Geometry check sheet. Reference: the model listing, model coordinates, mm. Face numbers are marked on the shaded views. A direction names the side the tool comes from. Give positions to 0.01 mm unless a question says otherwise; leave off trailing zeros. Write each loop counter-clockwise with the first axis right and the second up, starting at its lowest first coordinate (ties: lowest second). Pieces come first, ordered by that corner, then holes. Notation, with made-up numbers: M -25,51 L -13,51 A19 cw -13,58 Z; hole C -6.5,78.5 d5. An arc over 180 degrees is marked long. One line per item, written item: value. Start each with the question number.
1. Gauge pin test, flat ends, axial feed: pin 1 (3 mm diameter, centred on x = -74, z = -31.5, fed in from -Y); pin 2 (6 mm diameter, centred on x = -20, z = 45, fed in from +Y); pin 3 (6.5 mm diameter, centred on x = -40, z = 45.5, fed in from -Y); pin 4 (4 mm diameter, centred on x = 100, z = 45, fed in from +Y). Record the tip position at first contact, or that the pin passes through.
2. Cross-section at A-A on z = -45. Count the separate pieces of the cut face and the enclosed holes in it, then the cut area to 3 significant figures.
3. Cross-section at B-B on x = -51.5. Record the cut outline in (y, z).
4. Cross-section at C-C on z = 20. Record the cut outline in (x, y).
5. Tool access check on the marked faces 1 and 2. Record the directions out of +Z, -Z, +X, -X, +Y, -Y that give a thin tool (end or side, any length) a straight path to the whole face; none if there is none.
6. Release check for a two-part mould opening along Z. For the marked faces 3, 4 and 5 record: pulls with the +Z half, pulls with the -Z half, needs draft (parallel to the pull), parting line crosses it, or undercut.
7. Scan lines: line 1 (Z direction, x = -100, y = 9); line 2 (Z direction, x = 62, y = 9); line 3 (Z direction, x = 72.5, y = 7.5). Record each from-to range of solid material in increasing order.
from build123d import *

# Parameters (mm, degrees)
SKETCH2_W           = 240
SKETCH2_H           = 100
BOSS_EXTRUDE1_DEPTH = 12
HOLE1_AT_2_COUNT    = 2
HOLE1_AT_2_PITCH    = 228
SKETCH10_W          = 216
SKETCH10_H          = 76
CUT_EXTRUDE2_DEPTH  = 8
EXTRUDE_THIN1_DEPTH = 8
FILLET1_R           = 1


# Read off the part's stored shape, not the designer's step: CBORE for M4 SHCS1
with BuildPart() as part:
    # Sketch2 → Boss-Extrude1 (new body)
    with BuildSketch(Plane(origin=(0, 0, 0), x_dir=(1, 0, 0), z_dir=(0, 1, 0))):
        Rectangle(SKETCH2_W, SKETCH2_H)
    extrude(amount=BOSS_EXTRUDE1_DEPTH)

    # Sketch6 → Hole1 (revolve, cut)
    with BuildSketch(Plane(origin=(-114, 6, 50), x_dir=(0, -1, 0), z_dir=(1, 0, 0))):
        Polygon((0, 0), (0, 12), (1.85, 10.15), (1.85, 0), align=None)
    hole1 = revolve(axis=Axis((-114, 6, 54.244199587), (0, 0, -1)), mode=Mode.SUBTRACT)

    # Hole1 at 2: Hole1 ×2
    with Locations(*[(i * HOLE1_AT_2_PITCH, 0, 0) for i in range(1, HOLE1_AT_2_COUNT)]):
        add(hole1, mode=Mode.SUBTRACT)

    # Mirror2: Hole1 across plane
    add(hole1.mirror(Plane.XY), mode=Mode.SUBTRACT)

    # Mirror2 copy 1 sketch → Mirror2 copy 1 (revolve, cut)
    with BuildSketch(Plane(origin=(114, 6, -50), x_dir=(0, -1, 0), z_dir=(1, 0, 0))):
        Polygon((0, 0), (0, -12), (1.85, -10.15), (1.85, 0), align=None)
    revolve(axis=Axis((114, 6, -54.244199587), (0, 0, -1)), mode=Mode.SUBTRACT)

    # CBORE for M4 SHCS1 outline → CBORE for M4 SHCS1 (revolve, cut)
    with BuildSketch(Plane(origin=(-100, 0, -45), x_dir=(1, 0, 0), z_dir=(0, 0, 1))):
        Polygon((2.25, 4), (2.25, 12), (0, 12), (0, 0), (4.025, 0), (4, 0.025), (4, 4), align=None)
    revolve(axis=Axis((-100, 0, -45), (0, 1, 0)), mode=Mode.SUBTRACT)

    # CBORE for M4 SHCS1 2 outline → CBORE for M4 SHCS1 2 (revolve, cut)
    with BuildSketch(Plane(origin=(-100, 0, 45), x_dir=(1, 0, 0), z_dir=(0, 0, 1))):
        Polygon((0, 0), (4.025, 0), (4, 0.025), (4, 4), (2.25, 4), (2.25, 12), (0, 12), align=None)
    revolve(axis=Axis((-100, 0, 45), (0, 1, 0)), mode=Mode.SUBTRACT)

    # CBORE for M4 SHCS1 3 outline → CBORE for M4 SHCS1 3 (revolve, cut)
    with BuildSketch(Plane(origin=(-80, 0, -45), x_dir=(1, 0, 0), z_dir=(0, 0, 1))):
        Polygon((0, 0), (4.025, 0), (4, 0.025), (4, 4), (2.25, 4), (2.25, 12), (0, 12), align=None)
    revolve(axis=Axis((-80, 0, -45), (0, 1, 0)), mode=Mode.SUBTRACT)

    # CBORE for M4 SHCS1 4 outline → CBORE for M4 SHCS1 4 (revolve, cut)
    with BuildSketch(Plane(origin=(-80, 0, 45), x_dir=(1, 0, 0), z_dir=(0, 0, 1))):
        Polygon((0, 0), (4.025, 0), (4, 0.025), (4, 4), (2.25, 4), (2.25, 12), (0, 12), align=None)
    revolve(axis=Axis((-80, 0, 45), (0, 1, 0)), mode=Mode.SUBTRACT)

    # CBORE for M4 SHCS1 5 outline → CBORE for M4 SHCS1 5 (revolve, cut)
    with BuildSketch(Plane(origin=(-60, 0, -45), x_dir=(1, 0, 0), z_dir=(0, 0, 1))):
        Polygon((0, 0), (4.025, 0), (4, 0.025), (4, 4), (2.25, 4), (2.25, 12), (0, 12), align=None)
    revolve(axis=Axis((-60, 0, -45), (0, 1, 0)), mode=Mode.SUBTRACT)

    # CBORE for M4 SHCS1 6 outline → CBORE for M4 SHCS1 6 (revolve, cut)
    with BuildSketch(Plane(origin=(-60, 0, 45), x_dir=(1, 0, 0), z_dir=(0, 0, 1))):
        Polygon((0, 0), (4.025, 0), (4, 0.025), (4, 4), (2.25, 4), (2.25, 12), (0, 12), align=None)
    revolve(axis=Axis((-60, 0, 45), (0, 1, 0)), mode=Mode.SUBTRACT)

    # CBORE for M4 SHCS1 7 outline → CBORE for M4 SHCS1 7 (revolve, cut)
    with BuildSketch(Plane(origin=(-40, 0, -45), x_dir=(1, 0, 0), z_dir=(0, 0, 1))):
        Polygon((0, 0), (4.025, 0), (4, 0.025), (4, 4), (2.25, 4), (2.25, 12), (0, 12), align=None)
    revolve(axis=Axis((-40, 0, -45), (0, 1, 0)), mode=Mode.SUBTRACT)

    # CBORE for M4 SHCS1 8 outline → CBORE for M4 SHCS1 8 (revolve, cut)
    with BuildSketch(Plane(origin=(-40, 0, 45), x_dir=(1, 0, 0), z_dir=(0, 0, 1))):
        Polygon((0, 0), (4.025, 0), (4, 0.025), (4, 4), (2.25, 4), (2.25, 12), (0, 12), align=None)
    revolve(axis=Axis((-40, 0, 45), (0, 1, 0)), mode=Mode.SUBTRACT)

    # CBORE for M4 SHCS1 9 outline → CBORE for M4 SHCS1 9 (revolve, cut)
    with BuildSketch(Plane(origin=(-20, 0, -45), x_dir=(1, 0, 0), z_dir=(0, 0, 1))):
        Polygon((0, 0), (4.025, 0), (4, 0.025), (4, 4), (2.25, 4), (2.25, 12), (0, 12), align=None)
    revolve(axis=Axis((-20, 0, -45), (0, 1, 0)), mode=Mode.SUBTRACT)

    # CBORE for M4 SHCS1 10 outline → CBORE for M4 SHCS1 10 (revolve, cut)
    with BuildSketch(Plane(origin=(-20, 0, 45), x_dir=(1, 0, 0), z_dir=(0, 0, 1))):
        Polygon((0, 0), (4.025, 0), (4, 0.025), (4, 4), (2.25, 4), (2.25, 12), (0, 12), align=None)
    revolve(axis=Axis((-20, 0, 45), (0, 1, 0)), mode=Mode.SUBTRACT)

    # CBORE for M4 SHCS1 11 outline → CBORE for M4 SHCS1 11 (revolve, cut)
    with BuildSketch(Plane.XY.offset(-45)):
        Polygon((0, 0), (4.025, 0), (4, 0.025), (4, 4), (2.25, 4), (2.25, 12), (0, 12), align=None)
    revolve(axis=Axis((0, 0, -45), (0, 1, 0)), mode=Mode.SUBTRACT)

    # CBORE for M4 SHCS1 12 outline → CBORE for M4 SHCS1 12 (revolve, cut)
    with BuildSketch(Plane.XY.offset(45)):
        Polygon((0, 0), (4.025, 0), (4, 0.025), (4, 4), (2.25, 4), (2.25, 12), (0, 12), align=None)
    revolve(axis=Axis((0, 0, 45), (0, 1, 0)), mode=Mode.SUBTRACT)

    # CBORE for M4 SHCS1 13 outline → CBORE for M4 SHCS1 13 (revolve, cut)
    with BuildSketch(Plane(origin=(20, 0, -45), x_dir=(1, 0, 0), z_dir=(0, 0, 1))):
        Polygon((0, 0), (4.025, 0), (4, 0.025), (4, 4), (2.25, 4), (2.25, 12), (0, 12), align=None)
    revolve(axis=Axis((20, 0, -45), (0, 1, 0)), mode=Mode.SUBTRACT)

    # CBORE for M4 SHCS1 14 outline → CBORE for M4 SHCS1 14 (revolve, cut)
    with BuildSketch(Plane(origin=(20, 0, 45), x_dir=(1, 0, 0), z_dir=(0, 0, 1))):
        Polygon((0, 0), (4.025, 0), (4, 0.025), (4, 4), (2.25, 4), (2.25, 12), (0, 12), align=None)
    revolve(axis=Axis((20, 0, 45), (0, 1, 0)), mode=Mode.SUBTRACT)

    # CBORE for M4 SHCS1 15 outline → CBORE for M4 SHCS1 15 (revolve, cut)
    with BuildSketch(Plane(origin=(40, 0, -45), x_dir=(1, 0, 0), z_dir=(0, 0, 1))):
        Polygon((0, 0), (4.025, 0), (4, 0.025), (4, 4), (2.25, 4), (2.25, 12), (0, 12), align=None)
    revolve(axis=Axis((40, 0, -45), (0, 1, 0)), mode=Mode.SUBTRACT)

    # CBORE for M4 SHCS1 16 outline → CBORE for M4 SHCS1 16 (revolve, cut)
    with BuildSketch(Plane(origin=(40, 0, 45), x_dir=(1, 0, 0), z_dir=(0, 0, 1))):
        Polygon((0, 0), (4.025, 0), (4, 0.025), (4, 4), (2.25, 4), (2.25, 12), (0, 12), align=None)
    revolve(axis=Axis((40, 0, 45), (0, 1, 0)), mode=Mode.SUBTRACT)

    # CBORE for M4 SHCS1 17 outline → CBORE for M4 SHCS1 17 (revolve, cut)
    with BuildSketch(Plane(origin=(60, 0, -45), x_dir=(1, 0, 0), z_dir=(0, 0, 1))):
        Polygon((0, 0), (4.025, 0), (4, 0.025), (4, 4), (2.25, 4), (2.25, 12), (0, 12), align=None)
    revolve(axis=Axis((60, 0, -45), (0, 1, 0)), mode=Mode.SUBTRACT)

    # CBORE for M4 SHCS1 18 outline → CBORE for M4 SHCS1 18 (revolve, cut)
    with BuildSketch(Plane(origin=(60, 0, 45), x_dir=(1, 0, 0), z_dir=(0, 0, 1))):
        Polygon((0, 0), (4.025, 0), (4, 0.025), (4, 4), (2.25, 4), (2.25, 12), (0, 12), align=None)
    revolve(axis=Axis((60, 0, 45), (0, 1, 0)), mode=Mode.SUBTRACT)

    # CBORE for M4 SHCS1 19 outline → CBORE for M4 SHCS1 19 (revolve, cut)
    with BuildSketch(Plane(origin=(80, 0, -45), x_dir=(1, 0, 0), z_dir=(0, 0, 1))):
        Polygon((0, 0), (4.025, 0), (4, 0.025), (4, 4), (2.25, 4), (2.25, 12), (0, 12), align=None)
    revolve(axis=Axis((80, 0, -45), (0, 1, 0)), mode=Mode.SUBTRACT)

    # CBORE for M4 SHCS1 20 outline → CBORE for M4 SHCS1 20 (revolve, cut)
    with BuildSketch(Plane(origin=(80, 0, 45), x_dir=(1, 0, 0), z_dir=(0, 0, 1))):
        Polygon((0, 0), (4.025, 0), (4, 0.025), (4, 4), (2.25, 4), (2.25, 12), (0, 12), align=None)
    revolve(axis=Axis((80, 0, 45), (0, 1, 0)), mode=Mode.SUBTRACT)

    # CBORE for M4 SHCS1 21 outline → CBORE for M4 SHCS1 21 (revolve, cut)
    with BuildSketch(Plane(origin=(100, 0, -45), x_dir=(1, 0, 0), z_dir=(0, 0, 1))):
        Polygon((0, 0), (4.025, 0), (4, 0.025), (4, 4), (2.25, 4), (2.25, 12), (0, 12), align=None)
    revolve(axis=Axis((100, 0, -45), (0, 1, 0)), mode=Mode.SUBTRACT)

    # CBORE for M4 SHCS1 22 outline → CBORE for M4 SHCS1 22 (revolve, cut)
    with BuildSketch(Plane(origin=(100, 0, 45), x_dir=(1, 0, 0), z_dir=(0, 0, 1))):
        Polygon((0, 0), (4.025, 0), (4, 0.025), (4, 4), (2.25, 4), (2.25, 12), (0, 12), align=None)
    revolve(axis=Axis((100, 0, 45), (0, 1, 0)), mode=Mode.SUBTRACT)

    # Sketch10 → Cut-Extrude2 (cut)
    with BuildSketch(Plane.XZ):
        Rectangle(SKETCH10_W, SKETCH10_H)
    extrude(amount=-CUT_EXTRUDE2_DEPTH, mode=Mode.SUBTRACT)

    # Sketch11 → Extrude-Thin1 (add)
    with BuildSketch(Plane.XZ):
        Polygon((-107.336187577, -39.886624782), (108.663812423, 36.113375218), (107.336187577, 39.886624782), (-108.663812423, -36.113375218), align=None)
        Polygon((-108.663812423, 36.113375218), (107.336187577, -39.886624782), (108.663812423, -36.113375218), (-107.336187577, 39.886624782), align=None)
    extrude(amount=-EXTRUDE_THIN1_DEPTH)

    # Fillet1
    fillet1_edges = [part.edges().sort_by_distance(p)[0] for p in [
        (101.974201355, 4, 38),
        (6.025798645, 4, 0),
        (-108, 4, -35.879811588),
        (-6.025798645, 4, 0),
        (0, 4, -2.120188412),
        (108, 4, -35.879811588),
        (-101.974201355, 4, 38),
        (0, 4, 2.120188412),
        (108, 4, 35.879811588),
        (-101.974201355, 4, -38),
        (101.974201355, 4, -38),
        (-108, 4, 35.879811588),
    ]]
    fillet(fillet1_edges, radius=FILLET1_R)


solid = part.part
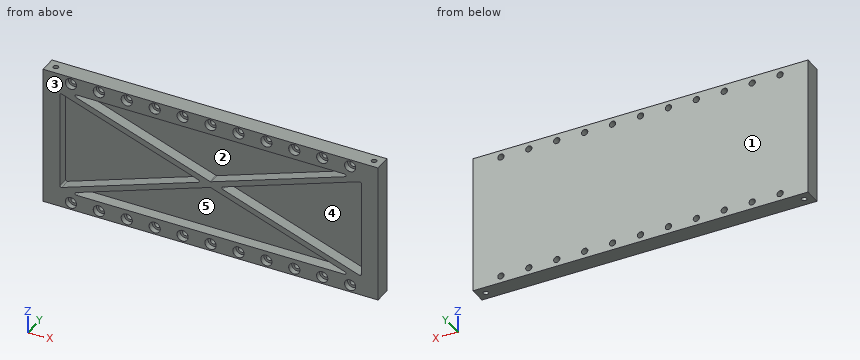
Report:
1. pin 1: stops at y = 8
1. pin 2: stops at y = 12
1. pin 3: stops at y = 4
1. pin 4: passes through
2. separate pieces: 12
2. enclosed holes: 2
2. area: 2,110 mm^2
3. outline: M 0,-50 L 12,-50 L 12,50 L 0,50 L 0,38 L 8,38 L 8,20.24 L 0,20.24 L 0,16 L 8,16 L 8,-16 L 0,-16 L 0,-20.24 L 8,-20.24 L 8,-38 L 0,-38 Z
4. outline: M -120,0 L -108,0 L -108,8 L -62.87,8 L -62.87,0 L -50.82,0 L -50.82,8 L 50.82,8 L 50.82,0 L 62.87,0 L 62.87,8 L 108,8 L 108,0 L 120,0 L 120,12 L -120,12 Z
5. face 1: +Z, -Z, +X, -X, +Y
5. face 2: -Y
6. face 3: needs draft
6. face 4: undercut
6. face 5: undercut
7. line 1: z = -50 to -47.25, -42.75 to 42.75, 47.25 to 50
7. line 2: z = -50 to -46.03, -43.97 to 43.97, 46.03 to 50
7. line 3: z = -50 to -38, -27.63 to -23.39, 23.39 to 27.63, 38 to 50
